Geometry check sheet. Reference: the model listing, model coordinates, mm. Face numbers are marked on the shaded views. A direction names the side the tool comes from. Give positions to 0.01 mm unless a question says otherwise; leave off trailing zeros. Write each loop counter-clockwise with the first axis right and the second up, starting at its lowest first coordinate (ties: lowest second). Pieces come first, ordered by that corner, then holes. Notation, with made-up numbers: (15.5, -5.75) - (66.5, -5.75) arc R33 ccw to (66.5, 26.25) - close; hole circle Ø11 at (-26, 86.25). An arc over 180 degrees is marked (long way). One line per question, with ' | ' between items. Start each with the question number.
Q1. Section check C-C on y = -24.5. Record the boundary of the cut face in (x, z).
Q2. Thickness scan on L1, parallel to Y at x = 0, z = 6.75; L2, parallel to Z at x = -0.25, y = -26; L3, parallel to Y at x = 2.25, z = 12.25. Record the ranges inside material, lowest first. Write a range as [from, to].
Q3. Section check A-A on x = 0.5. Record the boundary of the cut face in (y, z), and give its area (3 significant figures).
Q4. Section check D-D on z = 9. Record the boundary of the cut face in (x, y).
Q5. Section check B-B on z = 1.5. Record the boundary of the cut face in (x, y), and give its area (3 significant figures).
Q6. Gauge pin test, flat ends, axial feed: P1, Ø8, axis at y = -31, z = 9.5, coming from the -X side; P2, Ø4, axis at y = -39, z = 14.5, coming from the +X side; P3, Ø1, axis at x = 8, y = -30, coming from the -Z side; P4, Ø6, axis at x = -4.5, z = 14.5, coming from the +Y side. Record the tip position at first contact, or that the pin passes through.
Q7. Release check for a two-part mould opening along X. For the marked faces 3, 4 and 5 record: +X half, -X half, draft (parallel to the pull), parting line (faces both ways), or undercut.
Q8. Set-up check for the marked faces 1 and 2: record each of +Z, -Z, +X, -X, +Y, -Y from which the full face is reachable in a straight line by a thin tool's end or side.
```python
from build123d import *

# Parameters (mm, degrees)
SKETCH1_R           = 4
BOSS_EXTRUDE2_DEPTH = 18
SKETCH2_R           = 6.75
BOSS_EXTRUDE3_DEPTH = 35


with BuildPart() as part:
    # Sketch1 → Boss-Extrude2 (new body)
    with BuildSketch(Plane.XY):
        with BuildLine():
            Line((-9.75, 0), (-9.75, -17.25))
            Line((-9.75, -17.25), (9.75, -17.25))
            Line((9.75, -17.25), (9.75, 0))
            ThreePointArc((9.75, 0), (0, 9.75), (-9.75, 0))
        make_face()
        Circle(SKETCH1_R, mode=Mode.SUBTRACT)
    extrude(amount=BOSS_EXTRUDE2_DEPTH)

    # Sketch2 → Boss-Extrude3 (add)
    with BuildSketch(Plane.XZ.offset(17.25)):
        with Locations((0, 9)):
            Circle(SKETCH2_R)
    extrude(amount=BOSS_EXTRUDE3_DEPTH)


solid = part.part
```
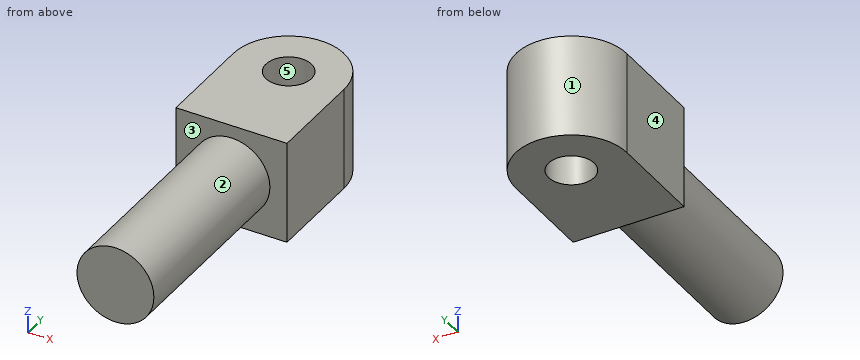
Working result:
1) outline: circle Ø13.5 at (0, 9)
2) L1: y = [-52.25, -4], [4, 9.75] | L2: z = [2.25, 15.75] | L3: y = [-52.25, -3.31], [3.31, 9.49]
3) outline: (-52.25, 2.27) - (-17.25, 2.27) - (-17.25, 0) - (-3.97, 0) - (-3.97, 18) - (-17.25, 18) - (-17.25, 15.73) - (-52.25, 15.73) - close; (3.97, 0) - (9.74, 0) - (9.74, 18) - (3.97, 18) - close | area: 814 mm2
4) outline: (-9.75, -17.25) - (-6.75, -17.25) - (-6.75, -52.25) - (6.75, -52.25) - (6.75, -17.25) - (9.75, -17.25) - (9.75, 0) arc R9.75 ccw to (-9.75, 0) - close; hole circle Ø8 at (0, 0)
5) outline: (-9.75, -17.25) - (9.75, -17.25) - (9.75, 0) arc R9.75 ccw to (-9.75, 0) - close; hole circle Ø8 at (0, 0) | area: 435 mm2
6) P1: stops at x = -6.75 | P2: stops at x = 5.77 | P3: passes through | P4: stops at y = 9.63
7) face 3: draft | face 4: -X half | face 5: undercut
8) face 1: +Z, -Z, +Y | face 2: -Y
